Here's how the part is built. I have some questions about the finished solid (model axes, mm). Give positions to 0.01 mm unless a question says otherwise; leave off trailing zeros. Loops run counter-clockwise (first coordinate to the right, second up) from the corner with the lowest first, then second, coordinate; pieces in that order, holes last. Notation, with made-up numbers: (-16, 11.25) - (39, 11.25) arc R15 ccw to (39, 28.25) - close; hole circle Ø1 at (15, -36.5). An arc over 180 degrees is marked (long way). Use a Markdown table: item, result.
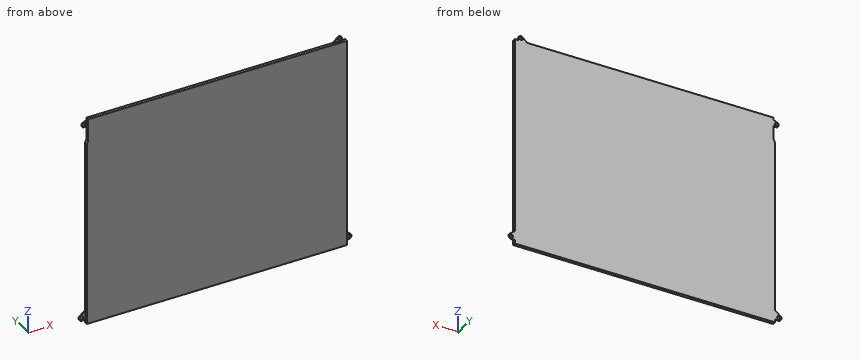
from build123d import *

# Parameters (mm, degrees)
F1_DEPTH = 2.5
F0_R     = 1.25
F2_DEPTH = 0.5
F3_W     = 200
F3_H     = 151
F4_DEPTH = 0.1


with BuildPart() as f1:
    # F0 (on Front) → F1 (new body)
    with BuildSketch(Plane.XZ):
        Polygon((-105, -83.83553), (105, -83.83553), (105, -80.83553), (105, -73.83553), (105, 84.16447), (102, 84.16447), (95, 84.16447), (-104, 84.16447), (-104, 82.16447), (-104, 77.16447), (-104, 66.16447), (-105, 64.16447), (-105, -73.83553), (-105, -81.33553), align=None)
    extrude(amount=F1_DEPTH)

    # F0 (on Front) → F2 (join)
    with BuildSketch(Plane.XZ):
        with BuildLine():
            Line((95, 84.16447), (102, 84.16447))
            Line((102, 84.16447), (102, 86.16447))
            ThreePointArc((102, 86.16447), (100.787839, 88.00276), (98.62069, 87.612746))
            Line((98.62069, 87.612746), (95, 84.16447))
        make_face()
        with Locations((100, 86.16447)):
            Circle(F0_R, mode=Mode.SUBTRACT)
        with BuildLine():
            Line((-106, 77.16447), (-104, 77.16447))
            Line((-104, 77.16447), (-104, 82.16447))
            Line((-104, 82.16447), (-106.769231, 81.010624))
            ThreePointArc((-106.769231, 81.010624), (-107.961161, 78.772238), (-106, 77.16447))
        make_face()
        with Locations((-106, 79.16447)):
            Circle(F0_R, mode=Mode.SUBTRACT)
        with BuildLine():
            Line((-108.040458, -81.33553), (-105, -81.33553))
            Line((-105, -81.33553), (-105, -73.83553))
            Line((-105, -73.83553), (-109.39797, -77.32289))
            ThreePointArc((-109.39797, -77.32289), (-110.131335, -79.806943), (-108.040458, -81.33553))
        make_face()
        with Locations((-108, -79.085893)):
            Circle(F0_R, mode=Mode.SUBTRACT)
        with BuildLine():
            Line((105, -73.83553), (105, -80.83553))
            Line((105, -80.83553), (107.329069, -80.83553))
            ThreePointArc((107.329069, -80.83553), (109.601422, -79.396099), (108.870329, -76.807459))
            Line((108.870329, -76.807459), (105, -73.83553))
        make_face()
        with Locations((107.5, -78.592032)):
            Circle(F0_R, mode=Mode.SUBTRACT)
    extrude(amount=F2_DEPTH)

    # F3 (on Front) → F4 (join)
    with BuildSketch(Plane.XZ):
        with Locations((-1, 0.66447)):
            Rectangle(F3_W, F3_H)
    extrude(amount=F4_DEPTH)


solid = f1.part
(1) If I drill on line 1 (Z direction, x = -106, y = -0.3); line 2 (X direction, y = -0.65, z = 21.5); line 3 (Z direction, x = -58, y = -0.55), over which ranges is the centre line in solid material (lowest first)?
A:
| item | result |
|---|---|
| line 1 | -81.34 to -74.63, 77.16 to 77.91, 80.41 to 81.33 |
| line 2 | -105 to 105 |
| line 3 | -83.84 to 84.16 |
(2) Suppose I cut it at C-C on z = -13. Write out the boundary of the cut face in (x, y), plus the area to 3 significant figures.
A:
| item | result |
|---|---|
| outline | (-105, -2.5) - (105, -2.5) - (105, 0) - (-105, 0) - close |
| area | 525 mm2 |
(3) Will these pins go through, and if not, where does the flat tip stop? pin 1 (2 mm diameter, centred on x = -106.5, z = 80, fed in from -Y); pin 2 (0.8 mm diameter, centred on y = -1, z = 77, fed in from -X).
A:
| item | result |
|---|---|
| pin 1 | y = -0.5 |
| pin 2 | x = -104 |
(4) Suppose I cut it at A-A on y = -1.6. Write out the boundary of the cut face in (x, z), plus the area to 3 significant figures.
A:
| item | result |
|---|---|
| outline | (-105, -83.84) - (105, -83.84) - (105, 84.16) - (-104, 84.16) - (-104, 66.16) - (-105, 64.16) - close |
| area | 35,300 mm2 |
(5) Suppose I cut it at B-B on x = 41. Write out the boundary of the cut face in (y, z), plus the area to 3 significant figures.
A:
| item | result |
|---|---|
| outline | (-2.5, -83.84) - (0, -83.84) - (0, 84.16) - (-2.5, 84.16) - close |
| area | 420 mm2 |
